CAD build for the part. Positions are in the model's coordinates, mm. A direction names the side the tool comes from. Round coordinates to 2 decimals unless told otherwise and drop trailing zeros. Write each loop counter-clockwise with the first axis right and the second up, starting at its lowest first coordinate (ties: lowest second). Pieces come first, ordered by that corner, then holes. Notation, with made-up numbers: (-40, 57) - (-32, 57) arc R17 ccw to (-32, 85) - close; hole circle Ø3 at (-21.5, 71.25). An arc over 180 degrees is marked (long way). Use one line per item in the form item = value. Start each with the question number.
Item 1: Drill centre lines: L1, parallel to X at y = 12, z = 3.25; L2, parallel to Z at x = 2, y = -10; L3, parallel to X at y = 35.5, z = 6.25. Where is each one in solid material? Low to high.
Item 2: Tool access for faces 1 (the flat face through (-12.5, -2, 4)), 2 (the flat face through (-13.5, -2, 4)), 3 (the flat face through (-5, -2, 0)): list every direction of +Z, -Z, +X, -X, +Y, -Y with a clear straight run to the whole face (end or side of a thin tool).
Item 3: Band-saw the part on A-A, the plane z = 4.25. List the corners of the cut face in (x, y).
Item 4: Pin check, flat tips, straight feed: pin 1 (0.5 mm diameter, centred on y = -122.5, z = 0.5, fed in from -X); pin 2 (0.5 mm diameter, centred on y = 122.5, z = 0.5, fed in from +X); pin 3 (1.1 mm diameter, centred on y = -101.5, z = 0.5, fed in from -X). Stop position of each tip, or through.
Item 5: Pull direction X, two halves, no side cores. Call faces 4 (the flat face through (16, -2, 6.501)), 5 (the flat face through (13.5, -2, 4)), 6 (the flat face through (12.5, -2, 4)): +X half, -X half, draft (parallel to the pull), parting line (faces both ways), or undercut.
Item 6: Band-saw the part on B-B, the plane y = 0. List the corners of the cut face in (x, z), and give its area (3 significant figures).
Item 7: Band-saw the part on C-C, the plane x = -6. List the corners of the cut face in (y, z).
from build123d import *

# Parameters (mm, degrees)
F1_DEPTH = 127
F3_DEPTH = 1.001
F4_DEPTH = 1


# Not quite as in the source:
# - a feature names something its author has since deleted; it is built from what else it names


with BuildPart() as f1:
    # F0 (on Front) → F1 (new body, symmetric)
    with BuildSketch(Plane.XZ):
        with BuildLine():
            ThreePointArc((-13.5001, 1.8), (-12.9728922061, 0.5272077939), (-11.7001, 0))
            Line((-11.7001, 0), (11.7001, 0))
            ThreePointArc((11.7001, 0), (12.9728922061, 0.5272077939), (13.5001, 1.8))
            Line((13.5001, 1.8), (13.5001, 5.70062))
            ThreePointArc((13.5001, 5.70062), (13.7344145751, 6.2663054249), (14.3001, 6.50062))
            Line((14.3001, 6.50062), (18.3269093243, 6.50062))
            Line((18.3269093243, 6.50062), (18.3269093243, 7.50062))
            Line((18.3269093243, 7.50062), (14.2999, 7.50062))
            ThreePointArc((14.2999, 7.50062), (13.0271077939, 6.9734122061), (12.4999, 5.70062))
            Line((12.4999, 5.70062), (12.4999, 1.8))
            ThreePointArc((12.4999, 1.8), (12.2655854249, 1.2343145751), (11.6999, 1))
            Line((11.6999, 1), (-11.7001, 1))
            ThreePointArc((-11.7001, 1), (-12.2657854249, 1.2343145751), (-12.5001, 1.8))
            Line((-12.5001, 1.8), (-12.5001, 5.70062))
            ThreePointArc((-12.5001, 5.70062), (-13.0273077939, 6.9734122061), (-14.3001, 7.50062))
            Line((-14.3001, 7.50062), (-16.6730906757, 7.50062))
            Line((-16.6730906757, 7.50062), (-16.6730906757, 6.50062))
            Line((-16.6730906757, 6.50062), (-14.3001, 6.50062))
            ThreePointArc((-14.3001, 6.50062), (-13.7344145751, 6.2663054249), (-13.5001, 5.70062))
            Line((-13.5001, 5.70062), (-13.5001, 1.8))
        make_face()
    extrude(amount=F1_DEPTH, both=True)

    # F2 (on face) → F3 (cut, through all)
    with BuildSketch(Plane.XY.offset(1)):
        with BuildLine():
            ThreePointArc((-3.1, -4.4), (0, -7.5), (3.1, -4.4))
            Line((3.1, -4.4), (3.1, 4.4))
            ThreePointArc((3.1, 4.4), (0, 7.5), (-3.1, 4.4))
            Line((-3.1, 4.4), (-3.1, -4.4))
        make_face()
        with BuildLine():
            ThreePointArc((-3.1, 20.6), (0, 17.5), (3.1, 20.6))
            Line((3.1, 20.6), (3.1, 29.4))
            ThreePointArc((3.1, 29.4), (0, 32.5), (-3.1, 29.4))
            Line((-3.1, 29.4), (-3.1, 20.6))
        make_face()
        with BuildLine():
            ThreePointArc((-3.1, 45.6), (0, 42.5), (3.1, 45.6))
            Line((3.1, 45.6), (3.1, 54.4))
            ThreePointArc((3.1, 54.4), (0, 57.5), (-3.1, 54.4))
            Line((-3.1, 54.4), (-3.1, 45.6))
        make_face()
        with BuildLine():
            ThreePointArc((-3.1, 70.6), (0, 67.5), (3.1, 70.6))
            Line((3.1, 70.6), (3.1, 79.4))
            ThreePointArc((3.1, 79.4), (0, 82.5), (-3.1, 79.4))
            Line((-3.1, 79.4), (-3.1, 70.6))
        make_face()
        with BuildLine():
            ThreePointArc((-3.1, 95.6), (0, 92.5), (3.1, 95.6))
            Line((3.1, 95.6), (3.1, 104.4))
            ThreePointArc((3.1, 104.4), (0, 107.5), (-3.1, 104.4))
            Line((-3.1, 104.4), (-3.1, 95.6))
        make_face()
        with BuildLine():
            ThreePointArc((-3.1, 120.6), (0, 117.5), (3.1, 120.6))
            Line((3.1, 120.6), (3.1, 129.4))
            ThreePointArc((3.1, 129.4), (0, 132.5), (-3.1, 129.4))
            Line((-3.1, 129.4), (-3.1, 120.6))
        make_face()
        with BuildLine():
            ThreePointArc((-3.1, -29.4), (0, -32.5), (3.1, -29.4))
            Line((3.1, -29.4), (3.1, -20.6))
            ThreePointArc((3.1, -20.6), (0, -17.5), (-3.1, -20.6))
            Line((-3.1, -20.6), (-3.1, -29.4))
        make_face()
        with BuildLine():
            ThreePointArc((3.1, -45.6), (0, -42.5), (-3.1, -45.6))
            Line((-3.1, -45.6), (-3.1, -54.4))
            ThreePointArc((-3.1, -54.4), (0, -57.5), (3.1, -54.4))
            Line((3.1, -54.4), (3.1, -45.6))
        make_face()
        with BuildLine():
            ThreePointArc((-3.1, -79.4), (0, -82.5), (3.1, -79.4))
            Line((3.1, -79.4), (3.1, -70.6))
            ThreePointArc((3.1, -70.6), (0, -67.5), (-3.1, -70.6))
            Line((-3.1, -70.6), (-3.1, -79.4))
        make_face()
        with BuildLine():
            ThreePointArc((3.1, -95.6), (0, -92.5), (-3.1, -95.6))
            Line((-3.1, -95.6), (-3.1, -104.4))
            ThreePointArc((-3.1, -104.4), (0, -107.5), (3.1, -104.4))
            Line((3.1, -104.4), (3.1, -95.6))
        make_face()
        with BuildLine():
            ThreePointArc((3.1, -120.6), (0, -117.5), (-3.1, -120.6))
            Line((-3.1, -120.6), (-3.1, -129.4))
            ThreePointArc((-3.1, -129.4), (0, -132.5), (3.1, -129.4))
            Line((3.1, -129.4), (3.1, -120.6))
        make_face()
    extrude(amount=-F3_DEPTH, mode=Mode.SUBTRACT)

    # F2 (on face) → F4 (cut, through all)
    with BuildSketch(Plane.XY.offset(1)):
        with BuildLine():
            ThreePointArc((-3.1, 95.6), (0, 92.5), (3.1, 95.6))
            Line((3.1, 95.6), (3.1, 104.4))
            ThreePointArc((3.1, 104.4), (0, 107.5), (-3.1, 104.4))
            Line((-3.1, 104.4), (-3.1, 95.6))
        make_face()
        with BuildLine():
            ThreePointArc((-3.1, 70.6), (0, 67.5), (3.1, 70.6))
            Line((3.1, 70.6), (3.1, 79.4))
            ThreePointArc((3.1, 79.4), (0, 82.5), (-3.1, 79.4))
            Line((-3.1, 79.4), (-3.1, 70.6))
        make_face()
        with BuildLine():
            ThreePointArc((-3.1, 45.6), (0, 42.5), (3.1, 45.6))
            Line((3.1, 45.6), (3.1, 54.4))
            ThreePointArc((3.1, 54.4), (0, 57.5), (-3.1, 54.4))
            Line((-3.1, 54.4), (-3.1, 45.6))
        make_face()
        with BuildLine():
            ThreePointArc((-3.1, 20.6), (0, 17.5), (3.1, 20.6))
            Line((3.1, 20.6), (3.1, 29.4))
            ThreePointArc((3.1, 29.4), (0, 32.5), (-3.1, 29.4))
            Line((-3.1, 29.4), (-3.1, 20.6))
        make_face()
        with BuildLine():
            ThreePointArc((-3.1, -4.4), (0, -7.5), (3.1, -4.4))
            Line((3.1, -4.4), (3.1, 4.4))
            ThreePointArc((3.1, 4.4), (0, 7.5), (-3.1, 4.4))
            Line((-3.1, 4.4), (-3.1, -4.4))
        make_face()
        with BuildLine():
            ThreePointArc((-3.1, 120.6), (0, 117.5), (3.1, 120.6))
            Line((3.1, 120.6), (3.1, 127))
            Line((3.1, 127), (-3.1, 127))
            Line((-3.1, 127), (-3.1, 120.6))
        make_face()
        with BuildLine():
            Line((-3.1, 127), (3.1, 127))
            Line((3.1, 127), (3.1, 129.4))
            ThreePointArc((3.1, 129.4), (0, 132.5), (-3.1, 129.4))
            Line((-3.1, 129.4), (-3.1, 127))
        make_face()
    extrude(amount=-F4_DEPTH, mode=Mode.SUBTRACT)


solid = f1.part
Determined:
q1.L1 = -13.5 to -12.5, 12.5 to 13.5
q1.L2 = 0 to 1
q1.L3 = -13.72 to -12.59, 12.59 to 13.72
q2.face_1 = +Z, +Y, -Y
q2.face_2 = -Z, -X, +Y, -Y
q2.face_3 = -Z, +X, -X, +Y, -Y
q3.outline = (-13.5, -127) - (-12.5, -127) - (-12.5, 127) - (-13.5, 127) - close; (12.5, -127) - (13.5, -127) - (13.5, 127) - (12.5, 127) - close
q4.pin_1 = -13.16
q4.pin_2 = 13.16
q4.pin_3 = -13.34
q5.face_4 = draft
q5.face_5 = +X half
q5.face_6 = undercut
q6.outline = (-16.67, 6.5) - (-14.3, 6.5) arc R0.8 cw to (-13.5, 5.7) - (-13.5, 1.8) arc R1.8 ccw to (-11.7, 0) - (-3.1, 0) - (-3.1, 1) - (-11.7, 1) arc R0.8 cw to (-12.5, 1.8) - (-12.5, 5.7) arc R1.8 ccw to (-14.3, 7.5) - (-16.67, 7.5) - close; (3.1, 0) - (11.7, 0) arc R1.8 ccw to (13.5, 1.8) - (13.5, 5.7) arc R0.8 cw to (14.3, 6.5) - (18.33, 6.5) - (18.33, 7.5) - (14.3, 7.5) arc R1.8 ccw to (12.5, 5.7) - (12.5, 1.8) arc R0.8 cw to (11.7, 1) - (3.1, 1) - close
q6.area = 39.6 mm²
q7.outline = (-127, 0) - (127, 0) - (127, 1) - (-127, 1) - close
